```python
from build123d import *

# Parameters (mm, degrees)
BOSS_EXTRUDE1_DEPTH       = 3
SKETCH2_W                 = 3.05
SKETCH2_H                 = 3.05
BOSS_EXTRUDE2_DEPTH       = 33
SKETCH3_W                 = 120
SKETCH3_H                 = 140
BOSS_EXTRUDE3_DEPTH       = 3
SKETCH4_W                 = 3.05
SKETCH4_H                 = 3.05
BOSS_EXTRUDE4_DEPTH       = 23
SKETCH6_W                 = 120
SKETCH6_H                 = 140
BOSS_EXTRUDE5_DEPTH       = 3
SKETCH7_W                 = 68
SKETCH7_H                 = 25
BOSS_EXTRUDE6_DEPTH       = 27
SKETCH9_W                 = 58
SKETCH9_H                 = 60
SKETCH9_W_2               = 20
SKETCH9_H_2               = 45
SKETCH9_W_3               = 30
SKETCH9_H_3               = 50
BOSS_EXTRUDE7_DEPTH       = 20
SKETCH10_W                = 53.46
SKETCH10_H                = 101.85
BOSS_EXTRUDE8_DEPTH       = 12
SKETCH11_W                = 110
SKETCH11_H                = 30
BOSS_EXTRUDE9_DEPTH       = 32
SKETCH12_W                = 140
SKETCH12_H                = 45
BOSS_EXTRUDE10_DEPTH      = 30
SKETCH13_W                = 20
SKETCH13_H                = 12.6
BOSS_EXTRUDE11_DEPTH      = 2.5
SKETCH14_W                = 3.6
SKETCH14_H                = 20
BOSS_EXTRUDE12_DEPTH      = 20
SKETCH15_W                = 3.6
SKETCH15_H                = 10
BOSS_EXTRUDE13_DEPTH      = 16
SKETCH16_W                = 3
SKETCH16_H                = 57
SKETCH16_H_2              = 25
BOSS_EXTRUDE14_DEPTH      = 50
BOSS_EXTRUDE15_DEPTH      = 23.4
BOSS_EXTRUDE15_DEPTH_BACK = 14.9
SKETCH17_W                = 39.808487161
SKETCH17_H                = 20
SKETCH18_W                = 78
SKETCH18_H                = 25
BOSS_EXTRUDE16_DEPTH      = 6


with BuildPart() as part:
    # Sketch1 → Boss-Extrude1 (new body)
    with BuildSketch(Plane(origin=(0, 0, 0), x_dir=(1, 0, 0), z_dir=(0, 1, 0))):
        Polygon((-73, -35), (-60, -19.801315846), (-60, 85), (60, 85), (60, -19.801315846), (73, -35), (73, -85), (60, -85), (-60, -85), (-73, -85), align=None)
    extrude(amount=BOSS_EXTRUDE1_DEPTH)

    # Sketch2 → Boss-Extrude2 (add)
    with BuildSketch(Plane(origin=(0, 3, 0), x_dir=(1, 0, 0), z_dir=(0, 1, 0))):
        with Locations((-53, -11.81)):
            Rectangle(SKETCH2_W, SKETCH2_H)
        with Locations((53, -11.81)):
            Rectangle(SKETCH2_W, SKETCH2_H)
        with Locations((54, 75)):
            Rectangle(SKETCH2_W, SKETCH2_H)
        with Locations((-54, 75)):
            Rectangle(SKETCH2_W, SKETCH2_H)
    extrude(amount=BOSS_EXTRUDE2_DEPTH)

    # Sketch3 → Boss-Extrude3 (add)
    with BuildSketch(Plane(origin=(0, 36, 0), x_dir=(1, 0, 0), z_dir=(0, 1, 0))):
        Polygon((-80, 74.780305915), (-60, 62.99), (-60, 122.99), (-80, 122.99), align=None)
        with Locations((0, 52.99)):
            Rectangle(SKETCH3_W, SKETCH3_H)
        Polygon((60, 122.99), (60, 62.99), (80, 74.780305915), (80, 122.99), align=None)
    extrude(amount=BOSS_EXTRUDE3_DEPTH)

    # Sketch4 → Boss-Extrude4 (add)
    with BuildSketch(Plane(origin=(0, 39, 0), x_dir=(1, 0, 0), z_dir=(0, 1, 0))):
        with Locations((-53, -11.81)):
            Rectangle(SKETCH4_W, SKETCH4_H)
        with Locations((-53, 116.99)):
            Rectangle(SKETCH4_W, SKETCH4_H)
        with Locations((53, -11.81)):
            Rectangle(SKETCH4_W, SKETCH4_H)
        with Locations((53, 116.99)):
            Rectangle(SKETCH4_W, SKETCH4_H)
    extrude(amount=BOSS_EXTRUDE4_DEPTH)

    # Sketch6 → Boss-Extrude5 (add)
    with BuildSketch(Plane(origin=(0, 62, 0), x_dir=(1, 0, 0), z_dir=(0, 1, 0))):
        with Locations((0, 52.99)):
            Rectangle(SKETCH6_W, SKETCH6_H)
    extrude(amount=BOSS_EXTRUDE5_DEPTH)

    # Sketch7 → Boss-Extrude6 (add)
    with BuildSketch(Plane.XZ.offset(-36)):
        with Locations((-46, -100.53)):
            Rectangle(SKETCH7_W, SKETCH7_H)
        with Locations((46, -100.53)):
            Rectangle(SKETCH7_W, SKETCH7_H)
    extrude(amount=BOSS_EXTRUDE6_DEPTH)

    # Sketch9 → Boss-Extrude7 (add)
    with BuildSketch(Plane(origin=(0, 39, 0), x_dir=(1, 0, 0), z_dir=(0, 1, 0))):
        with Locations((-1.05, 85.88)):
            Rectangle(SKETCH9_W, SKETCH9_H)
        with Locations((-35.64, 8.98)):
            Rectangle(SKETCH9_W_2, SKETCH9_H_2)
        with Locations((35.64, 8.98)):
            Rectangle(SKETCH9_W_2, SKETCH9_H_2)
        with Locations((0, 11.48)):
            Rectangle(SKETCH9_W_3, SKETCH9_H_3)
    extrude(amount=BOSS_EXTRUDE7_DEPTH)

    # Sketch10 → Boss-Extrude8 (add)
    with BuildSketch(Plane(origin=(0, 65, 0), x_dir=(1, 0, 0), z_dir=(0, 1, 0))):
        with Locations((-0.81, 72.065)):
            Rectangle(SKETCH10_W, SKETCH10_H)
    extrude(amount=BOSS_EXTRUDE8_DEPTH)

    # Sketch11 → Boss-Extrude9 (add)
    with BuildSketch(Plane(origin=(0, 3, 0), x_dir=(1, 0, 0), z_dir=(0, 1, 0))):
        with Locations((0, 7.543684861)):
            Rectangle(SKETCH11_W, SKETCH11_H)
    extrude(amount=BOSS_EXTRUDE9_DEPTH)

    # Sketch12 → Boss-Extrude10 (add)
    with BuildSketch(Plane(origin=(0, 3, 0), x_dir=(1, 0, 0), z_dir=(0, 1, 0))):
        with Locations((0, 47.793183731)):
            Rectangle(SKETCH12_W, SKETCH12_H)
    extrude(amount=BOSS_EXTRUDE10_DEPTH)

    # Sketch13 → Boss-Extrude11 (add)
    with BuildSketch(Plane(origin=(0, 65, 0), x_dir=(1, 0, 0), z_dir=(0, 1, 0))):
        with Locations((31.68, -6.09)):
            Rectangle(SKETCH13_W, SKETCH13_H)
    extrude(amount=BOSS_EXTRUDE11_DEPTH)

    # Sketch14 → Boss-Extrude12 (add)
    with BuildSketch(Plane(origin=(0, 39, 0), x_dir=(1, 0, 0), z_dir=(0, 1, 0))):
        with Locations((54.75, 37.99)):
            Rectangle(SKETCH14_W, SKETCH14_H)
        with Locations((-54.75, 37.99)):
            Rectangle(SKETCH14_W, SKETCH14_H)
    extrude(amount=BOSS_EXTRUDE12_DEPTH)

    # Sketch15 → Boss-Extrude13 (add)
    with BuildSketch(Plane(origin=(0, 3, 0), x_dir=(1, 0, 0), z_dir=(0, 1, 0))):
        with Locations((72.3, -72)):
            Rectangle(SKETCH15_W, SKETCH15_H)
        with Locations((-72.3, -72)):
            Rectangle(SKETCH15_W, SKETCH15_H)
    extrude(amount=BOSS_EXTRUDE13_DEPTH)

    # Sketch16 → Boss-Extrude14 (add)
    with BuildSketch(Plane(origin=(0, 3, 0), x_dir=(1, 0, 0), z_dir=(0, 1, 0))):
        with Locations((55.5, -46.6)):
            Rectangle(SKETCH16_W, SKETCH16_H)
        with Locations((-56.5, -58.5)):
            Rectangle(SKETCH16_W, SKETCH16_H_2)
    extrude(amount=BOSS_EXTRUDE14_DEPTH)

    # Sketch17 → Boss-Extrude15 (add, two sides: drawn at the far end of the back side and taken through both)
    with BuildSketch(Plane(origin=(57, 0, 0), x_dir=(0, 0, -1), z_dir=(1, 0, 0)).offset(-BOSS_EXTRUDE15_DEPTH_BACK)):
        with Locations((-46.50705122, 35)):
            Rectangle(SKETCH17_W, SKETCH17_H)
    extrude(amount=BOSS_EXTRUDE15_DEPTH + BOSS_EXTRUDE15_DEPTH_BACK)

    # Sketch18 → Boss-Extrude16 (add)
    with BuildSketch(Plane.XZ):
        with Locations((0, 78.5)):
            Rectangle(SKETCH18_W, SKETCH18_H)
    extrude(amount=BOSS_EXTRUDE16_DEPTH)


solid = part.part
```
Can you work these out from the model? Positions are in its coordinate system, mm. A direction names the side the tool comes from. Round coordinates to 2 decimals unless told otherwise and drop trailing zeros. Order: outer loops, then holes, each group sorted by start corner. A loop starts at its lowest first (then second) coordinate and runs counter-clockwise, first axis right, second up.
(1) On a 3-axis mill with a long thin cutter (end or side, diameter ignored), from which of +Z, -Z, +X, -X, +Y, -Y can I reach the whole of each face in a straight line? I mean faces 1 (the face through (-46, 23, -113.03)), 2 (the face through (-74.1, 11, 72)), 3 (the face through (-25.64, 49, -9)), 4 (the face through (56.55, 49, -38)), 5 (the face through (-36, 49, -31.48)). Say none if no direction works.
Results are:
face 1: -Z, +X, -X, -Y
face 2: +Z, -X, +Y, -Y
face 3: +Z
face 4: -Z, +X
face 5: none
(2) If we section it at B-B (z = -95): Please give me the cut outline in (x, y).
Results are:
outline: (-80, 9) - (-12, 9) - (-12, 36) - (12, 36) - (12, 9) - (80, 9) - (80, 39) - (27.95, 39) - (27.95, 59) - (-30.05, 59) - (-30.05, 39) - (-80, 39) - close; (-60, 62) - (60, 62) - (60, 65) - (25.92, 65) - (25.92, 77) - (-27.54, 77) - (-27.54, 65) - (-60, 65) - close
(3) If I drill on L1, parallel to Z at x = 66, y = 26.5; L2, parallel to Y at x = 7, z = -45; L3, parallel to X at y = 48, z = 4, over which ranges is the centre line in solid material (lowest first)?
Results are:
L1: z = -113.03 to -88.03, -70.29 to -25.29, 26.6 to 66.41
L2: y = 0 to 33, 36 to 39, 62 to 77
L3: x = -45.64 to -25.64, -15 to 15, 25.64 to 45.64
(4) If we section it at A-A (x = -34.5): Count the separate pieces of the cut face and the enclosed holes in it, plus the area to 4 significant figures.
Results are:
separate pieces: 3
enclosed holes: 0
area: 5,385 mm2
(5) I'm going to push flat-ended pins straight in: pin 1 (4 mm diameter, centred on x = -54, y = 51, fed in from -Z) (3 decimals); pin 2 (3.5 mm diameter, centred on y = 45.5, z = -117, fed in from -X) (3 decimals); pin 3 (10 mm diameter, centred on x = 2, z = 13, fed in from +Y); pin 4 (10 mm diameter, centred on y = 35, z = 23, fed in from +X). Where does each tip first touch, or does it pass through?
Results are:
pin 1: stops at z = -118.515
pin 2: stops at x = -54.525
pin 3: stops at y = 65
pin 4: stops at x = 80.4
(6) We'd pull the mould along Z, two halves only. Please class faces 6 (the face through (-66.591, 1.479, 27.507)), 7 (the face through (-1, 49, -55.88)), 8 (the face through (-1, 18, -25.293)), 9 (the face through (-15, 49, -11)): +Z half, -Z half, draft (parallel to the pull), parting line (faces both ways), or undercut.
Results are:
face 6: -Z half
face 7: undercut
face 8: undercut
face 9: draft
(7) If we section it at C-C (z = -8.5): Please give me the cut outline in (x, y).
Results are:
outline: (-60, 0) - (60, 0) - (60, 3) - (55, 3) - (55, 35) - (-55, 35) - (-55, 3) - (-60, 3) - close; (-60, 36) - (60, 36) - (60, 39) - (45.64, 39) - (45.64, 59) - (25.64, 59) - (25.64, 39) - (15, 39) - (15, 59) - (-15, 59) - (-15, 39) - (-25.64, 39) - (-25.64, 59) - (-45.64, 59) - (-45.64, 39) - (-60, 39) - close; (-60, 62) - (60, 62) - (60, 65) - (-60, 65) - close
